Could you check a few things on this model? Use its own coordinates, in mm. Give positions to 0.01 mm unless a question says otherwise; leave off trailing zeros. Loops run counter-clockwise (first coordinate to the right, second up) from the corner with the lowest first, then second, coordinate; pieces in that order, holes last. Notation, with made-up numbers: (21, -17) - (35, -17) arc R8 ccw to (35, -7) - close; hole circle Ø7 at (8, 26.5). An arc over 180 degrees is marked (long way). Answer in a Markdown table with one row per item. Add a question column.
```python
from build123d import *

# Parameters (mm, degrees)
BOSS_EXTRUDE1_DEPTH = 5
SKETCH2_R           = 5
CUT_EXTRUDE1_DEPTH  = 35
SKETCH3_W           = 40
SKETCH3_H           = 38
CUT_EXTRUDE2_DEPTH  = 35


with BuildPart() as part:
    # Sketch1 → Boss-Extrude1 (new body)
    with BuildSketch(Plane.XY):
        with BuildLine():
            Line((10, 0), (180, 0))
            ThreePointArc((180, 0), (187.071067812, 2.928932188), (190, 10))
            Line((190, 10), (190, 100))
            ThreePointArc((190, 100), (187.071067812, 107.071067812), (180, 110))
            Line((180, 110), (10, 110))
            ThreePointArc((10, 110), (2.928932188, 107.071067812), (0, 100))
            Line((0, 100), (0, 10))
            ThreePointArc((0, 10), (2.928932188, 2.928932188), (10, 0))
        make_face()
    extrude(amount=BOSS_EXTRUDE1_DEPTH)

    # Sketch2 → Cut-Extrude1 (cut)
    with BuildSketch(Plane(origin=(0, 0, 0), x_dir=(-1, 0, 0), z_dir=(0, 0, -1))):
        with Locations((-180, 100)):
            Circle(SKETCH2_R)
        with Locations((-10, 100)):
            Circle(SKETCH2_R)
        with Locations((-180, 10)):
            Circle(SKETCH2_R)
        with Locations((-10, 10)):
            Circle(SKETCH2_R)
    extrude(amount=-CUT_EXTRUDE1_DEPTH, mode=Mode.SUBTRACT)

    # Sketch3 → Cut-Extrude2 (cut)
    with BuildSketch(Plane.XY.offset(5)):
        with Locations((49.464961526, 73.72693734)):
            Rectangle(SKETCH3_W, SKETCH3_H)
    extrude(amount=-CUT_EXTRUDE2_DEPTH, mode=Mode.SUBTRACT)


solid = part.part
```
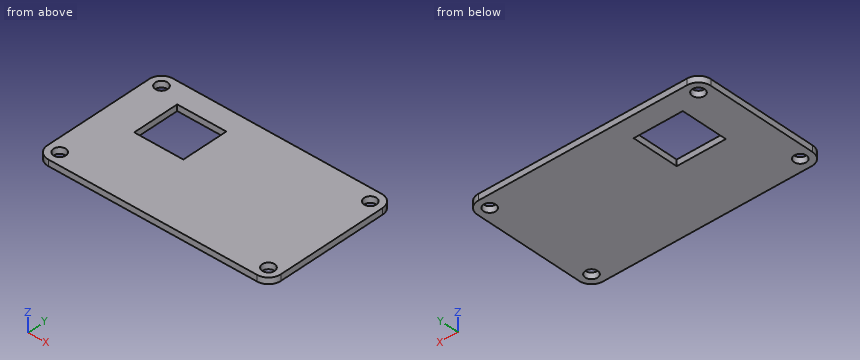
(1) I want a section at A-A on y = 72. Please give me the cut outline in (x, z), then the cut area to 3 significant figures.
(2) I want a section at C-C on z = 2.95. Please give me the cut outline in (x, y), then the cut area to 3 significant figures.
(3) Please list where these lines run through material, in increasing order: line 1 (Y direction, x = 10, z = 2.55); line 2 (X direction, y = 55, z = 4.25); line 3 (Y direction, x = 58.5, z = 4.3).
(4) I want a section at B-B on x = 63.5. Please give me the cut outline in (y, z).
Reported:
| question | item | result |
|---|---|---|
| 1 | outline | (0, 0) - (29.46, 0) - (29.46, 5) - (0, 5) - close; (69.46, 0) - (190, 0) - (190, 5) - (69.46, 5) - close |
| 1 | area | 750 mm² |
| 2 | outline | (0, 10) arc R10 ccw to (10, 0) - (180, 0) arc R10 ccw to (190, 10) - (190, 100) arc R10 ccw to (180, 110) - (10, 110) arc R10 ccw to (0, 100) - close; hole circle Ø10 at (10, 10); hole circle Ø10 at (10, 100); hole (29.46, 54.73) - (69.46, 54.73) - (69.46, 92.73) - (29.46, 92.73) - close; hole circle Ø10 at (180, 10); hole circle Ø10 at (180, 100) |
| 2 | area | 19,000 mm² |
| 3 | line 1 | 0 to 5, 15 to 95, 105 to 110 |
| 3 | line 2 | 0 to 29.46, 69.46 to 190 |
| 3 | line 3 | 0 to 54.73, 92.73 to 110 |
| 4 | outline | (0, 0) - (54.73, 0) - (54.73, 5) - (0, 5) - close; (92.73, 0) - (110, 0) - (110, 5) - (92.73, 5) - close |
